Part model, mm, in its own coordinate system. A direction names the side the tool comes from. Coordinates: 2 decimals unless noted, no trailing zeros. Loops run counter-clockwise (first coordinate to the right, second up) from the corner with the lowest first, then second, coordinate; pieces in that order, holes last. Notation, with made-up numbers: (19.25, 10) -> (72.25, 10) arc R34 cw to (72.25, 44) -> close; hole circle Ø1 at (65, 61.5). An arc over 180 degrees is marked (long way). Use one line per item in the form item = value. Start each with the question number.
(1) Mould opens along Y. For faces 1 (the cylindrical face through (-4.336, -42.605, 90.476)), 2 (the flat face through (-1, 35, 88)), 3 (the conical face through (-95.15, 4.19, 0.24)) say: +Y half, -Y half, draft (parallel to the pull), parting line (faces both ways), or undercut.
(2) Pin check, flat tips, straight feed: P1, Ø1.5, axis at y = -48.5, z = 10.5, coming from the +X side; P2, Ø10, axis at x = 40.5, z = 82, coming from the -Y side; P3, Ø21, axis at x = 16.5, y = -6, coming from the +Z side. Stop position of each tip, or through.
(3) Band-saw the part on B-B on y = 0. Give the cut face in (x, z).
(4) Drill centre lines: L1, parallel to Y at x = -27, z = 146.5; L2, parallel to Z at x = 0, y = 45; L3, parallel to Y at x = -1, z = -19.5. Where is each one in solid material? Low to high. Write a range as [from, to].
(5) 3-axis set-ups, long thin cutter, end or side, ignore diameter. For faces 4 (the flat face through (50, 3, 58)), 5 (the flat face through (-50, -0.7, 59.6)), 6 (the flat face through (-11.8, -50, 93.5)): which of +Z, -Z, +X, -X, +Y, -Y reach the whole face in a straight line?
(6) Band-saw the part on A-A on x = 0. Give the cut face in (y, z).
(7) Band-saw the part on C-C on z = -5.5. Give the cut face in (x, y).
```python
from build123d import *

# Parameters (mm, degrees)
SKETCH_R        = 100
PAD_DEPTH       = 50
CHAMFER_SIZE    = 5
SKETCH001_R     = 38
PAD001_DEPTH    = 50
SKETCH002_W     = 100
SKETCH002_H     = 100
PAD002_DEPTH    = 10
PAD003_DEPTH    = 50
SKETCH004_R     = 20
POCKET_DEPTH    = 101
SKETCH005_W     = 100
SKETCH005_H     = 101
POCKET001_DEPTH = 35


with BuildPart() as part:
    # Sketch → Pad (new body)
    with BuildSketch(Plane.XY):
        Circle(SKETCH_R)
    extrude(amount=PAD_DEPTH)

    # Chamfer
    chamfer_edges = [part.edges().sort_by_distance(p)[0] for p in [
        (-100, 0, 0),
    ]]
    chamfer(chamfer_edges, length=CHAMFER_SIZE)

    # Sketch001 (on Face4 of Chamfer) → Pad001 (join)
    with BuildSketch(Plane(origin=(0, 0, 0), x_dir=(1, 0, 0), z_dir=(0, 0, -1))):
        Circle(SKETCH001_R)
    extrude(amount=PAD001_DEPTH)

    # Sketch002 (on Face3 of Pad001) → Pad002 (join)
    with BuildSketch(Plane.XY.offset(50)):
        Rectangle(SKETCH002_W, SKETCH002_H)
    extrude(amount=PAD002_DEPTH)

    # Sketch003 → Pad003 (join, symmetric)
    with BuildSketch(Plane.XZ):
        with BuildLine():
            ThreePointArc((50, 110), (0, 160), (-50, 110))
            Line((-50, 60), (-50, 110))
            Line((50, 60), (-50, 60))
            Line((50, 110), (50, 60))
        make_face()
    extrude(amount=PAD003_DEPTH, both=True)

    # Sketch004 (on Face11 of Pad003) → Pocket (cut)
    with BuildSketch(Plane.XZ.offset(50)):
        with Locations((0, 110)):
            Circle(SKETCH004_R)
    extrude(amount=-POCKET_DEPTH, mode=Mode.SUBTRACT)

    # Sketch005 → Pocket001 (cut, symmetric)
    with BuildSketch(Plane.XZ):
        with Locations((0, 110.5)):
            Rectangle(SKETCH005_W, SKETCH005_H)
    extrude(amount=POCKET001_DEPTH, both=True, mode=Mode.SUBTRACT)


solid = part.part
```
A:
q1.face_1 = draft
q1.face_2 = undercut
q1.face_3 = parting line
q2.P1 = 87.86
q2.P2 = -50
q2.P3 = 60
q3.outline = (-100, 5) -> (-95, 0) -> (-38, 0) -> (-38, -50) -> (38, -50) -> (38, 0) -> (95, 0) -> (100, 5) -> (100, 50) -> (50, 50) -> (50, 60) -> (-50, 60) -> (-50, 50) -> (-100, 50) -> close
q4.L1 = [-50, -35], [35, 50]
q4.L2 = [0, 90], [130, 160]
q4.L3 = [-37.99, 37.99]
q5.face_4 = +Z, +X, +Y, -Y
q5.face_5 = +Z, -X, +Y, -Y
q5.face_6 = +Z, +X, -X, -Y
q6.outline = (-100, 5) -> (-95, 0) -> (-38, 0) -> (-38, -50) -> (38, -50) -> (38, 0) -> (95, 0) -> (100, 5) -> (100, 50) -> (50, 50) -> (50, 90) -> (35, 90) -> (35, 60) -> (-35, 60) -> (-35, 90) -> (-50, 90) -> (-50, 50) -> (-100, 50) -> close; (-50, 130) -> (-35, 130) -> (-35, 160) -> (-50, 160) -> close; (35, 130) -> (50, 130) -> (50, 160) -> (35, 160) -> close
q7.outline = circle Ø76 at (0, 0)
